from build123d import *

# Parameters (mm, degrees)
F0_W     = 889
F0_H     = 177.8
F0_R     = 2.7813
F1_DEPTH = 1.27


with BuildPart() as f1:
    # F0 (on Front) → F1 (new body)
    with BuildSketch(Plane.XZ):
        Rectangle(F0_W, F0_H)
        with Locations((-311.15, -66.675)):
            Circle(F0_R, mode=Mode.SUBTRACT)
        with Locations((-120.65, -66.675)):
            Circle(F0_R, mode=Mode.SUBTRACT)
        with BuildLine():
            Line((-381, 50.8), (-50.8, 50.8))
            ThreePointArc((-50.8, 50.8), (-46.309872, 48.940128), (-44.45, 44.45))
            Line((-44.45, 44.45), (-44.45, -44.45))
            ThreePointArc((-44.45, -44.45), (-46.309872, -48.940128), (-50.8, -50.8))
            Line((-50.8, -50.8), (-381, -50.8))
            ThreePointArc((-381, -50.8), (-385.490128, -48.940128), (-387.35, -44.45))
            Line((-387.35, -44.45), (-387.35, 44.45))
            ThreePointArc((-387.35, 44.45), (-385.490128, 48.940128), (-381, 50.8))
        make_face(mode=Mode.SUBTRACT)
        with Locations((-311.15, 66.675)):
            Circle(F0_R, mode=Mode.SUBTRACT)
        with Locations((-120.65, 66.675)):
            Circle(F0_R, mode=Mode.SUBTRACT)
    extrude(amount=F1_DEPTH)


solid = f1.part
The model under review builds one solid part; all positions refer to its coordinate system, in mm. Coordinates: 2 decimals unless noted, no trailing zeros. Write each loop counter-clockwise with the first axis right and the second up, starting at its lowest first coordinate (ties: lowest second). Pieces come first, ordered by that corner, then holes. Notation, with made-up numbers: (-1, 8.5) - (5, 8.5) arc R17 cw to (5, 36.5) - close; hole circle Ø9 at (29, -8). An arc over 180 degrees is marked (long way). Answer as CSV lines item,"result".
(1) We need section A-A (z = -30). Give the boundary of the cut face in (x, y), plus the area to 3 significant figures.
Data:
outline,"(-444.5, -1.27) - (-387.35, -1.27) - (-387.35, 0) - (-444.5, 0) - close; (-44.45, -1.27) - (444.5, -1.27) - (444.5, 0) - (-44.45, 0) - close"
area,"694 mm2"
(2) For line 1 along Z through (x, y) = (-120.65, -0.5); line 2 along Z through (x, y) = (-188, -0.8); line 3 along X through (y, z) = (-0.3, -39), list the stretches that pass through material, from the lowest coordinate up. Write a range as [from, to].
Data:
line 1,"z = [-88.9, -69.46], [-63.89, -50.8], [50.8, 63.89], [69.46, 88.9]"
line 2,"z = [-88.9, -50.8], [50.8, 88.9]"
line 3,"x = [-444.5, -387.35], [-44.45, 444.5]"
(3) We need section B-B (x = -70.5). Give the boundary of the cut face in (y, z), plus the area to 3 significant figures.
Data:
outline,"(-1.27, -88.9) - (0, -88.9) - (0, -50.8) - (-1.27, -50.8) - close; (-1.27, 50.8) - (0, 50.8) - (0, 88.9) - (-1.27, 88.9) - close"
area,"96.8 mm2"
(4) We need section C-C (y = -0.9). Give the boundary of the cut face in (x, z) (3 decimals).
Data:
outline,"(-444.5, -88.9) - (444.5, -88.9) - (444.5, 88.9) - (-444.5, 88.9) - close; hole (-387.35, -44.45) arc R6.35 ccw to (-381, -50.8) - (-50.8, -50.8) arc R6.35 ccw to (-44.45, -44.45) - (-44.45, 44.45) arc R6.35 ccw to (-50.8, 50.8) - (-381, 50.8) arc R6.35 ccw to (-387.35, 44.45) - close; hole circle Ø5.563 at (-311.15, -66.675); hole circle Ø5.563 at (-311.15, 66.675); hole circle Ø5.563 at (-120.65, -66.675); hole circle Ø5.563 at (-120.65, 66.675)"
